```python
from build123d import *

# Parameters (mm, degrees)
CROQUIS2_W              = 92.3
CROQUIS2_H              = 25.3
SALIENTE_EXTRUIR1_DEPTH = 12
VACIADO1_T              = -2.5
CROQUIS3_R              = 4
CROQUIS3_R_2            = 2
CORTAR_EXTRUIR1_DEPTH   = 12
SALIENTE_EXTRUIR2_START = 9.5
CROQUIS5_R              = 4
SALIENTE_EXTRUIR2_DEPTH = 9.5


with BuildPart() as part:
    # Croquis2 → Saliente-Extruir1 (new body)
    with BuildSketch(Plane.XY):
        with Locations((46.15, 12.65)):
            Rectangle(CROQUIS2_W, CROQUIS2_H)
    extrude(amount=SALIENTE_EXTRUIR1_DEPTH)

    # Vaciado1
    vaciado1_openings = [part.faces().sort_by_distance(p)[0] for p in [
        (46.15, 12.65, 12),
    ]]
    offset(amount=VACIADO1_T, openings=vaciado1_openings, kind=Kind.INTERSECTION)

    # Croquis3 → Cortar-Extruir1 (cut)
    with BuildSketch(Plane.XY.offset(2.5)):
        with Locations((46.15, 12.65)):
            Circle(CROQUIS3_R)
        with Locations((12.65, 12.65)):
            Circle(CROQUIS3_R_2)
        with Locations((79.65, 12.65)):
            Circle(CROQUIS3_R_2)
    extrude(amount=-CORTAR_EXTRUIR1_DEPTH, mode=Mode.SUBTRACT)

    # Croquis5 → Saliente-Extruir2 (add)
    with BuildSketch(Plane.XY.offset(2.5).offset(SALIENTE_EXTRUIR2_START)):
        with BuildLine():
            Line((28.65, 2.5), (63.65, 2.5))
            ThreePointArc((63.65, 2.5), (57.258552241, 6.60889898), (52.65, 12.65))
            ThreePointArc((52.65, 12.65), (46.15, 19.15), (39.65, 12.65))
            ThreePointArc((39.65, 12.65), (35.041447759, 6.60889898), (28.65, 2.5))
        make_face()
        with Locations(Location((46.15, 12.65, 0), (0, 0, 180))):
            Circle(CROQUIS5_R, mode=Mode.SUBTRACT)
    extrude(amount=-SALIENTE_EXTRUIR2_DEPTH)


solid = part.part
```
Source: CAD feature listing. Evaluate the final solid. Frame: model axes, mm. A direction names the side the tool comes from. Coordinates: 2 decimals unless noted, no trailing zeros. Loops run counter-clockwise (first coordinate to the right, second up) from the corner with the lowest first, then second, coordinate; pieces in that order, holes last. Notation, with made-up numbers: M -15,26 L 15,26 A36 ccw 15,60 Z; hole C -29.75,-7 d5. An arc over 180 degrees is marked long. Use CSV: the item, a comma, the result in double quotes.
(1) Cut plane C-C on y = 21.5. Return loops of the section in (x, z), and give its area (3 significant figures).
Answers follow:
outline,"M 0,0 L 92.3,0 L 92.3,12 L 89.8,12 L 89.8,2.5 L 2.5,2.5 L 2.5,12 L 0,12 Z"
area,"278 mm²"
(2) Line query: line 1 (Y direction, x = 11, z = 10); line 2 (Y direction, x = 79.65, z = 1.5); line 3 (X direction, y = 3, z = 11.75). Output: solid intervals per line, ascending. Write a range as [from, to].
Answers follow:
line 1,"[0, 2.5], [22.8, 25.3]"
line 2,"[0, 10.65], [14.65, 25.3]"
line 3,"[0, 2.5], [29.75, 62.55], [89.8, 92.3]"
(3) Cut plane D-D on x = 79.65. Return loops of the section in (y, z), and give its area (3 significant figures).
Answers follow:
outline,"M 0,0 L 10.65,0 L 10.65,2.5 L 2.5,2.5 L 2.5,12 L 0,12 Z; M 14.65,0 L 25.3,0 L 25.3,12 L 22.8,12 L 22.8,2.5 L 14.65,2.5 Z"
area,"101 mm²"
(4) Cut plane A-A on z = 10.25. Return loops of the section in (x, y).
Answers follow:
outline,"M 0,0 L 92.3,0 L 92.3,25.3 L 0,25.3 Z; hole M 2.5,2.5 L 28.65,2.5 A21.96 ccw 39.65,12.65 A6.5 cw 52.65,12.65 A21.96 ccw 63.65,2.5 L 89.8,2.5 L 89.8,22.8 L 2.5,22.8 Z; hole C 46.15,12.65 d8"
(5) Reachability of faces 4 (the face through (46, 0, 6)), 5 (the face through (46, 20, 2.5)) from +Z, -Z, +X, -X, +Y, -Y: full face, straight path, thin tool, end or side. Return the list, or none.
Answers follow:
face 4,"+Z, -Z, +X, -X, -Y"
face 5,"+Z"
(6) Draft query along X for faces 1 (the face through (92.3, 12, 6)), 2 (the face through (46, 25.3, 6)), 3 (the face through (15, 2.5, 7)). Return one class per face: pulls with the +X half, pulls with the -X half, needs draft (parallel to the pull), parting line crosses it, or undercut.
Answers follow:
face 1,"pulls with the +X half"
face 2,"needs draft"
face 3,"undercut"
(7) Contact query for flat-ended pins moving along their axis: pin 1 (1 mm diameter, centred on x = 12, y = 17, fed in from +Z); pin 2 (1.5 mm diameter, centred on x = 41, z = 10.5, fed in from -Y); pin 3 (6.5 mm diameter, centred on x = 46.15, y = 12.65, fed in from +Z). Output: stop coordinate, or through.
Answers follow:
pin 1,"z = 2.5"
pin 2,"y = 0"
pin 3,"through"
(8) Cut plane B-B on x = 46.15. Return loops of the section in (y, z).
Answers follow:
outline,"M 0,0 L 8.65,0 L 8.65,12 L 0,12 Z; M 16.65,0 L 25.3,0 L 25.3,12 L 22.8,12 L 22.8,2.5 L 19.15,2.5 L 19.15,12 L 16.65,12 Z"
